from build123d import *

# Parameters (mm, degrees)
F0_W     = 399
F0_H     = 256
F0_W_2   = 393.4
F0_H_2   = 250.4
F1_DEPTH = 1.5
F2_SIZE  = 1
F3_F1_R  = 1
F3_F2_R  = 1
F3_F3_R  = 1
F3_F4_R  = 1
F3_F5_R  = 1
F3_F6_R  = 1
F3_F7_R  = 1
F3_F8_R  = 1


with BuildPart() as f1:
    # F0 (on Top) → F1 (new body, symmetric)
    with BuildSketch(Plane.XY):
        Rectangle(F0_W, F0_H)
        Rectangle(F0_W_2, F0_H_2, mode=Mode.SUBTRACT)
    extrude(amount=F1_DEPTH, both=True)

    # F2
    f2_edges = [f1.edges().sort_by_distance(p)[0] for p in [
        (0, -128, 1.5),
        (-199.5, 0, 1.5),
        (0, 128, 1.5),
        (199.5, 0, 1.5),
    ]]
    chamfer(f2_edges, length=F2_SIZE)

    # F3: fillet of radius 1 on 8 edges, made by hand

    # F3_f1
    f3_f1_edges = [f1.edges().sort_by_distance(p)[0] for p in [
        (199.5, 128, -0.5),
    ]]
    fillet(f3_f1_edges, radius=F3_F1_R)

    # F3_f2
    f3_f2_edges = [f1.edges().sort_by_distance(p)[0] for p in [
        (199.5, -128, -0.5),
    ]]
    fillet(f3_f2_edges, radius=F3_F2_R)

    # F3_f3
    f3_f3_edges = [f1.edges().sort_by_distance(p)[0] for p in [
        (-199.5, 128, -0.5),
    ]]
    fillet(f3_f3_edges, radius=F3_F3_R)

    # F3_f4
    f3_f4_edges = [f1.edges().sort_by_distance(p)[0] for p in [
        (198.8535533906, -127.3535533906, 1.1464466094),
    ]]
    fillet(f3_f4_edges, radius=F3_F4_R)

    # F3_f5
    f3_f5_edges = [f1.edges().sort_by_distance(p)[0] for p in [
        (198.8535533906, 127.3535533906, 1.1464466094),
    ]]
    fillet(f3_f5_edges, radius=F3_F5_R)

    # F3_f6
    f3_f6_edges = [f1.edges().sort_by_distance(p)[0] for p in [
        (-199.5, -128, -0.5),
    ]]
    fillet(f3_f6_edges, radius=F3_F6_R)

    # F3_f7
    f3_f7_edges = [f1.edges().sort_by_distance(p)[0] for p in [
        (-198.8535533906, 127.3535533906, 1.1464466094),
    ]]
    fillet(f3_f7_edges, radius=F3_F7_R)

    # F3_f8
    f3_f8_edges = [f1.edges().sort_by_distance(p)[0] for p in [
        (-198.8535533906, -127.3535533906, 1.1464466094),
    ]]
    fillet(f3_f8_edges, radius=F3_F8_R)


solid = f1.part
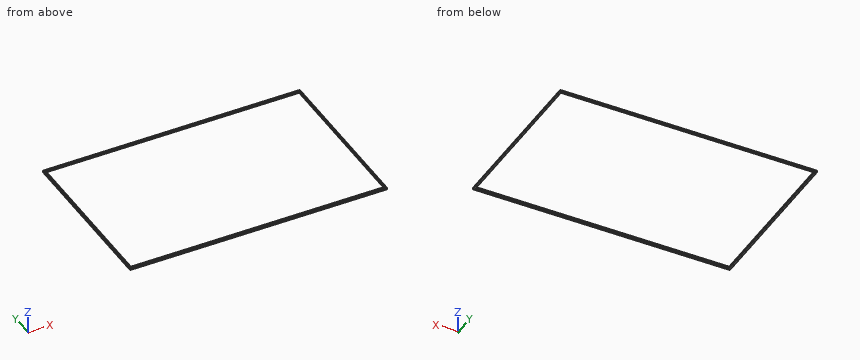
Input: part model. Units: mm. Frame: model coordinates. Round coordinates to 2 decimals unless told otherwise and drop trailing zeros. Loops run counter-clockwise (first coordinate to the right, second up) from the corner with the lowest first, then second, coordinate; pieces in that order, holes last. Notation, with made-up numbers: (-9.75, 18.5) -> (8.25, 18.5) arc R18 ccw to (8.25, 42.5) -> close; hole circle Ø5 at (84, 29). An arc over 180 degrees is marked (long way). Answer as a JSON object with one key per item and string values. Group by question number.
1) Section query B-B on z = -0.4. Output: boundary loops of the cut face in (x, y).
2) Section query C-C on y = 73.5. Output: boundary loops of the cut face in (x, z).
3) Ray query, L1, parallel to Y at x = 32, z = -0.95; L2, parallel to X at y = 109, z = 0.4; L3, parallel to X at y = 33.5, z = 0.6. Return the intervals inside material, ascending.
4) Section query A-A on x = -153.5. Output: boundary loops of the cut face in (y, z), plus the area to 3 significant figures.
Reply:
{
 "1": {"outline": "(-199.5, -127) arc R1 ccw to (-198.5, -128) -> (198.5, -128) arc R1 ccw to (199.5, -127) -> (199.5, 127) arc R1 ccw to (198.5, 128) -> (-198.5, 128) arc R1 ccw to (-199.5, 127) -> close; hole (-196.7, -125.2) -> (196.7, -125.2) -> (196.7, 125.2) -> (-196.7, 125.2) -> close"},
 "2": {"outline": "(-199.5, -1.5) -> (-196.7, -1.5) -> (-196.7, 1.5) -> (-198.5, 1.5) -> (-199.5, 0.5) -> close; (196.7, -1.5) -> (199.5, -1.5) -> (199.5, 0.5) -> (198.5, 1.5) -> (196.7, 1.5) -> close"},
 "3": {"L1": "y = -128 to -125.2, 125.2 to 128", "L2": "x = -199.5 to -196.7, 196.7 to 199.5", "L3": "x = -199.4 to -196.7, 196.7 to 199.4"},
 "4": {"outline": "(-128, -1.5) -> (-125.2, -1.5) -> (-125.2, 1.5) -> (-127, 1.5) -> (-128, 0.5) -> close; (125.2, -1.5) -> (128, -1.5) -> (128, 0.5) -> (127, 1.5) -> (125.2, 1.5) -> close", "area": "15.8 mm2"}
}
